Autodesk Inventor part; units mm, degrees
ref_plane "YZ Plane" through (0, 0, 0) normal (1, 0, 0) x (0, 1, 0)
ref_plane "XZ Plane" through (0, 0, 0) normal (0, 1, 0) x (-1, 0, 0)
ref_plane "XY Plane" through (0, 0, 0) normal (0, 0, 1) x (1, 0, 0)
sketch "Sketch1" plane through (0, 0, 0) normal (0, 1, 0) x (-1, 0, 0)
  circle A0 centre (0, 0) radius 18
  circle A1 centre (8, -8) radius 2.06
  circle A2 centre (8, 8) radius 2.06
  circle A3 centre (-8, 8) radius 2.06
  circle A4 centre (-8, -8) radius 2.06
  dimension "d0" = 36
  dimension "d1" = 4.12
  dimension "d2" = 8
  dimension "d3" = 8
  dimension "d6" = 360
extrude "Extrusion1" add sketch "Sketch1" along normal blind 6
properties part number "EndEffector_Stage1BearingClamp"
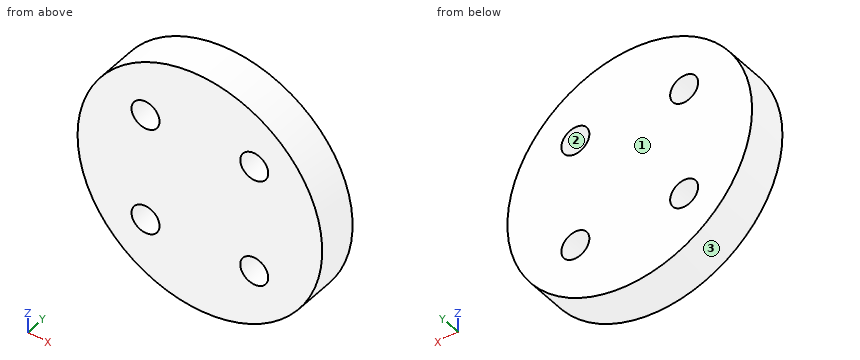
Source: CAD feature listing. Evaluate the final solid. Frame: model axes, mm. Face numbers are marked on the shaded views. Coordinates: 2 decimals unless noted, no trailing zeros. Loops run counter-clockwise (first coordinate to the right, second up) from the corner with the lowest first, then second, coordinate; pieces in that order, holes last. Notation, with made-up numbers: M -15.75,76.25 L -7.75,76.25 A29 ccw -7.75,103.25 Z; hole C 8,23 d5. An arc over 180 degrees is marked long. Use a Markdown table: item, result. Add a question column.
Q1. Section query C-C, the plane x = 8.5. Return loops of the section in (y, z).
Q2. Section query A-A, the plane y = 4.3. Return loops of the section in (x, z), and give its area (3 significant figures).
Q3. Section query B-B, the plane z = 8. Return loops of the section in (x, y), and give its area (3 significant figures).
Q4. First-contact query: pin 1 (6.5 mm diameter, centred on x = -8, z = 8, fed in from -Y); pin 2 (2.5 mm diameter, centred on x = -8, z = -8, fed in from +Y). Flat tips, straight axial feed; report the tip coordinate or a pass-through.
Q5. Draft query along Z for the marked faces 1, 2 and 3. Return one class per face: pulls with the +Z half, pulls with the -Z half, needs draft (parallel to the pull), parting line crosses it, or undercut.
Q6. Section query D-D, the plane z = 12.5. Return loops of the section in (x, y).
Q7. Material intervals for L1, parallel to X at y = 2.9, z = -7.5; L2, parallel to Z at x = -8, y = 4; L3, parallel to X at y = 3.5, z = 6.5, sorted ascending.
Result:
| question | item | result |
|---|---|---|
| 1 | outline | M 0,-15.87 L 6,-15.87 L 6,-10 L 0,-10 Z; M 0,-6 L 6,-6 L 6,6 L 0,6 Z; M 0,10 L 6,10 L 6,15.87 L 0,15.87 Z |
| 2 | outline | C 0,0 d36; hole C -8,-8 d4.12; hole C -8,8 d4.12; hole C 8,-8 d4.12; hole C 8,8 d4.12 |
| 2 | area | 965 mm2 |
| 3 | outline | M -16.12,0 L -10.06,0 L -10.06,6 L -16.12,6 Z; M -5.94,0 L 5.94,0 L 5.94,6 L -5.94,6 Z; M 10.06,0 L 16.12,0 L 16.12,6 L 10.06,6 Z |
| 3 | area | 144 mm2 |
| 4 | pin 1 | stops at y = 0 |
| 4 | pin 2 | passes through |
| 5 | face 1 | needs draft |
| 5 | face 2 | undercut |
| 5 | face 3 | parting line crosses it |
| 6 | outline | M -12.95,0 L 12.95,0 L 12.95,6 L -12.95,6 Z |
| 7 | L1 | x = -16.36 to -10, -6 to 6, 10 to 16.36 |
| 7 | L2 | z = -16.12 to -10.06, -5.94 to 5.94, 10.06 to 16.12 |
| 7 | L3 | x = -16.79 to -9.41, -6.59 to 6.59, 9.41 to 16.79 |
